from build123d import *

# Parameters (mm, degrees)
F0_W     = 1000
F0_H     = 450
F0_W_2   = 250
F0_H_2   = 410
F0_W_3   = 420
F1_DEPTH = 200
F2_W     = 400
F2_H     = 20
F3_DEPTH = 420


# Not quite as in the source:
# - a feature names something its author has since deleted; it is built from what else it names


with BuildPart() as f1:
    # F0 (on Front) → F1 (new body, symmetric)
    with BuildSketch(Plane.XZ):
        Rectangle(F0_W, F0_H)
        with Locations((-355, 0)):
            Rectangle(F0_W_2, F0_H_2, mode=Mode.SUBTRACT)
        Rectangle(F0_W_3, F0_H_2, mode=Mode.SUBTRACT)
        with Locations((355, 0)):
            Rectangle(F0_W_2, F0_H_2, mode=Mode.SUBTRACT)
    extrude(amount=F1_DEPTH, both=True)

    # F2 (on face) → F3 (join, through all)
    with BuildSketch(Plane(origin=(210, 0, 0), x_dir=(0, -1, 0), z_dir=(-1, 0, 0))):
        Rectangle(F2_W, F2_H)
    extrude(amount=F3_DEPTH)


solid = f1.part
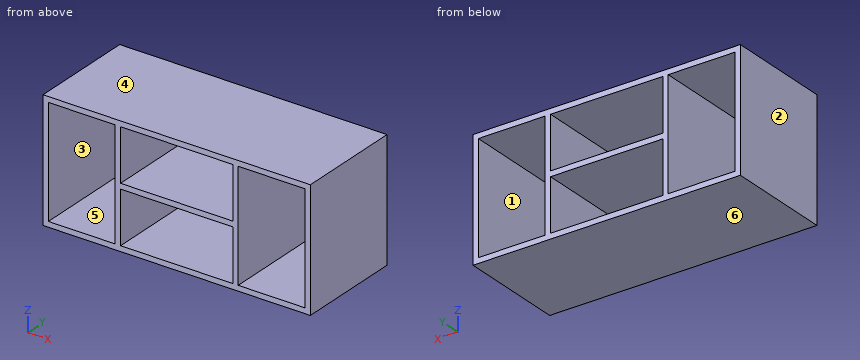
Work out the finished part from the listing and answer in its coordinate system (mm). Face numbers are marked on the shaded views. A direction names the side the tool comes from. Round coordinates to 2 decimals unless told otherwise and drop trailing zeros. Order: outer loops, then holes, each group sorted by start corner. A loop starts at its lowest first (then second) coordinate and runs counter-clockwise, first axis right, second up. Notation, with made-up numbers: M 13.25,11.5 L 20.25,11.5 A31 ccw 20.25,48.5 Z; hole C 33,87 d11. An arc over 180 degrees is marked long. Put each result on its own line as item: value. Start each with the question number.
Q1. For a pull along Z with two mould halves and no side action, classify the marked faces 3, 4, 5 and 6 as pulls with the +Z half, pulls with the -Z half, needs draft (parallel to the pull), parting line crosses it, or undercut.
Q2. Section C-C, the plane x = -46.5 is taken. Write down the section's boundary in (y, z), and give its area (3 significant figures).
Q3. Section D-D, the plane y = 160.5 is taken. Write down the section's boundary in (x, z), and give its area (3 significant figures).
Q4. Section B-B, the plane z = -43 is taken. Write down the section's boundary in (x, y), and give its area (3 significant figures).
Q5. A tool of negligible diameter and unlimited length cuts with its end or side. For the marked faces 1 and 2, from which of +Z, -Z, +X, -X, +Y, -Y can it reach the whole face along a straight path? Write none if from no direction.
Q6. Section A-A, the plane x = -320 is taken. Write down the section's boundary in (y, z), and give its area (3 significant figures).
Q7. Straight lines are drawn through the part: L1, parallel to X at y = 125, z = 105; L2, parallel to Z at x = 116, y = -38; L3, parallel to Z at x = 450.5, y = -131.5. For each, find the intervals that lie inside material, in ascending order. Write a range as [from, to].
Findings below:
1. face 3: undercut
1. face 4: pulls with the +Z half
1. face 5: undercut
1. face 6: pulls with the -Z half
2. outline: M -200,-225 L 200,-225 L 200,-205 L -200,-205 Z; M -200,-10 L 200,-10 L 200,10 L -200,10 Z; M -200,205 L 200,205 L 200,225 L -200,225 Z
2. area: 24,000 mm^2
3. outline: M -500,-225 L 500,-225 L 500,225 L -500,225 Z; hole M -480,-205 L -230,-205 L -230,205 L -480,205 Z; hole M -210,-205 L 210,-205 L 210,-10 L -210,-10 Z; hole M -210,10 L 210,10 L 210,205 L -210,205 Z; hole M 230,-205 L 480,-205 L 480,205 L 230,205 Z
3. area: 81,200 mm^2
4. outline: M -500,-200 L -480,-200 L -480,200 L -500,200 Z; M -230,-200 L -210,-200 L -210,200 L -230,200 Z; M 210,-200 L 230,-200 L 230,200 L 210,200 Z; M 480,-200 L 500,-200 L 500,200 L 480,200 Z
4. area: 32,000 mm^2
5. face 1: +Y, -Y
5. face 2: +Z, -Z, -X, +Y, -Y
6. outline: M -200,-225 L 200,-225 L 200,-205 L -200,-205 Z; M -200,205 L 200,205 L 200,225 L -200,225 Z
6. area: 16,000 mm^2
7. L1: x = [-500, -480], [-230, -210], [210, 230], [480, 500]
7. L2: z = [-225, -205], [-10, 10], [205, 225]
7. L3: z = [-225, -205], [205, 225]
